For this review, take the finished solid that the model builds, in its own axes (mm). A direction names the side the tool comes from. Coordinates: 2 decimals unless noted, no trailing zeros. Write each loop counter-clockwise with the first axis right and the second up, starting at its lowest first coordinate (ties: lowest second). Pieces come first, ordered by that corner, then holes. Notation, with made-up numbers: M 15.25,-18 L 51.25,-18 A23 cw 51.25,11 Z; hole C 1,11 d2. An arc over 180 degrees is marked long. One line per question, with ' | ' between items.
from build123d import *

# Parameters (mm, degrees)
F0_W     = 89.253187
F0_H     = 60.325
F1_DEPTH = 1.905
F3_DEPTH = 6.35
F5_DEPTH = 25.4
F6_W     = 53.34
F6_H     = 7.62
F7_DEPTH = 25.4


# Not quite as in the source:
# - a feature names something its author has since deleted; it is built from what else it names


with BuildPart() as f1:
    # F0 (on Top) → F1 (new body)
    with BuildSketch(Plane.XY):
        Rectangle(F0_W, F0_H)
    extrude(amount=F1_DEPTH)

    # F2 (on face) → F3 (join)
    with BuildSketch(Plane(origin=(0, 0, 0), x_dir=(1, 0, 0), z_dir=(0, 0, -1))):
        Polygon((-42.7215935, -28.2575), (-42.7215935, 28.2575), (44.6265935, 28.2575), (44.6265935, 30.1625), (-44.6265935, 30.1625), (-44.6265935, -30.1625), (44.6265935, -30.1625), (44.6265935, -28.2575), align=None)
    extrude(amount=F3_DEPTH)

    # F4 (on face) → F5 (cut)
    with BuildSketch(Plane.XZ.offset(30.1625)):
        with BuildLine():
            Line((-37.0065935, -5.842), (-37.0065935, -6.35))
            Line((-37.0065935, -6.35), (-26.8465935, -6.35))
            Line((-26.8465935, -6.35), (-26.8465935, -5.842))
            ThreePointArc((-26.8465935, -5.842), (-26.9953832552, -5.4827897552), (-27.3545935, -5.334))
            Line((-27.3545935, -5.334), (-36.4985935, -5.334))
            ThreePointArc((-36.4985935, -5.334), (-36.8578037448, -5.4827897552), (-37.0065935, -5.842))
        make_face()
        with BuildLine():
            Line((-19.4805935, -4.699), (-19.4805935, -6.35))
            Line((-19.4805935, -6.35), (-1.7005935, -6.35))
            Line((-1.7005935, -6.35), (-1.7005935, -4.699))
            ThreePointArc((-1.7005935, -4.699), (-2.4445422758, -2.9029487758), (-4.2405935, -2.159))
            Line((-4.2405935, -2.159), (-16.9405935, -2.159))
            ThreePointArc((-16.9405935, -2.159), (-18.7366447242, -2.9029487758), (-19.4805935, -4.699))
        make_face()
        with BuildLine():
            Line((6.8084065, -4.699), (6.8084065, -6.35))
            Line((6.8084065, -6.35), (15.1904065, -6.35))
            Line((15.1904065, -6.35), (15.1904065, -4.699))
            ThreePointArc((15.1904065, -4.699), (14.4464577242, -2.9029487758), (12.6504065, -2.159))
            Line((12.6504065, -2.159), (9.3484065, -2.159))
            ThreePointArc((9.3484065, -2.159), (7.5523552758, -2.9029487758), (6.8084065, -4.699))
        make_face()
    extrude(amount=-F5_DEPTH, mode=Mode.SUBTRACT)

    # F6 (on face) → F7 (cut)
    with BuildSketch(Plane.XY.offset(1.905)):
        with Locations((-10.0825935, 24.4475)):
            Rectangle(F6_W, F6_H)
    extrude(amount=-F7_DEPTH, mode=Mode.SUBTRACT)


solid = f1.part
1) The part is to be moulded in two halves that separate along X. For faces 6 (the flat face through (-44.627, 0, -2)), 7 (the cylindrical face through (7.572, -29.223, -2.883)), 8 (the flat face through (-1, 0, 1.905)), say which applies: +X half, -X half, draft (parallel to the pull), parting line (faces both ways), or undercut.
Responses:
face 6: -X half | face 7: undercut | face 8: draft
2) To check wall thickness, follow line 1 along Y through (x, z) = (-6, 1); line 2 along Y through (x, z) = (22, -4); line 3 along Y through (x, z) = (11.5, -5.75). State the ranges of each line that lie inside material, in increasing order. Write a range as [from, to].
Responses:
line 1: [-30.16, 20.64], [28.26, 30.16] | line 2: [-30.16, -28.26], [28.26, 30.16] | line 3: [28.26, 30.16]
3) Machinability: for faces 1 (the flat face through (-23, -29, -6.35)), 2 (the flat face through (16.587, 24, 1)), 3 (the flat face through (2, 28.258, -2)), 4 (the flat face through (-42.722, 0, -3)), 5 (the flat face through (-11, -29, -2.159)), which of the approach directions +Z, -Z, +X, -X, +Y, -Y give a long, thin tool a straight path to every point of the face, cutting with its end or side? Answer none if there is none.
Responses:
face 1: -Z, +X, -X, +Y, -Y | face 2: +Z, -Z | face 3: -Z | face 4: -Z, +X | face 5: -Z, -Y
4) Insertion check: pin 1 Ø1 at (x, y) = (10.5, -29.5) entering from -Z; pin 2 Ø3 at (y, z) = (2, -3.5) entering from +X. Each pin has a flat end and moves straight along its axis. Give the tip position at first contact, or say it passes through.
Responses:
pin 1: z = -2.16 | pin 2: x = -42.72
5) We need section B-B on y = 12.5. State the section outline as (x, z) points (3 decimals).
Responses:
outline: M -44.627,-6.35 L -42.722,-6.35 L -42.722,0 L 44.627,0 L 44.627,1.905 L -44.627,1.905 Z
